For this review, take the finished solid that the model builds, in its own axes (mm). A direction names the side the tool comes from. Give positions to 0.01 mm unless a question says otherwise; leave off trailing zeros. Order: outer loops, then holes, each group sorted by start corner. A loop starts at its lowest first (then second) coordinate and runs counter-clockwise, first axis right, second up. Notation, with made-up numbers: (-33, 79) - (-21, 79) arc R10 cw to (-21, 93) - close; hole circle Ø10 at (21.5, 8). An arc over 180 degrees is marked (long way). Answer as a JSON object with one key per item and string values. Group by question number.
from build123d import *

# Parameters (mm, degrees)
BOSS_EXTRUDE1_DEPTH   = 3
SKETCH2_R             = 6
BOSS_EXTRUDE2_DEPTH   = 4
SKETCH3_R             = 5
BOSS_EXTRUDE3_DEPTH   = 6
SKETCH4_R             = 2.6
CUT_EXTRUDE1_DEPTH    = 20.474342094
SKETCH5_R             = 4
CUT_EXTRUDE2_DEPTH    = 2.5
CUT_EXTRUDE3_START    = -3
SKETCH6_R             = 4
CUT_EXTRUDE3_DEPTH    = 3
M3X0_5_TAPPED_HOLE1_D = 2.5
CHAMFER1_SIZE         = 0.2
FILLET1_R             = 1


with BuildPart() as part:
    # Sketch1 → Boss-Extrude1 (new body)
    with BuildSketch(Plane(origin=(0, 0, 0), x_dir=(1, 0, 0), z_dir=(0, 1, 0))):
        with BuildLine():
            ThreePointArc((-2.104162541, 6.15), (-4.71280541, 4.47654612), (-6.25, 1.785357107))
            ThreePointArc((-6.25, 1.785357107), (-10.5, 0), (-6.25, -1.785357107))
            ThreePointArc((-6.25, -1.785357107), (-4.71280541, -4.47654612), (-2.104162541, -6.15))
            ThreePointArc((-2.104162541, -6.15), (0, -10), (2.104162541, -6.15))
            ThreePointArc((2.104162541, -6.15), (4.71280541, -4.47654612), (6.25, -1.785357107))
            ThreePointArc((6.25, -1.785357107), (10.5, 0), (6.25, 1.785357107))
            ThreePointArc((6.25, 1.785357107), (4.71280541, 4.47654612), (2.104162541, 6.15))
            ThreePointArc((2.104162541, 6.15), (0, 10), (-2.104162541, 6.15))
        make_face()
    extrude(amount=BOSS_EXTRUDE1_DEPTH)

    # Sketch2 → Boss-Extrude2 (add)
    with BuildSketch(Plane(origin=(0, 3, 0), x_dir=(1, 0, 0), z_dir=(0, 1, 0))):
        with Locations(Location((0, 0, 0), (0, 0, 270))):
            Circle(SKETCH2_R)
    extrude(amount=BOSS_EXTRUDE2_DEPTH)

    # Sketch3 → Boss-Extrude3 (add)
    with BuildSketch(Plane(origin=(0, 7, 0), x_dir=(1, 0, 0), z_dir=(0, 1, 0))):
        with Locations(Location((0, 0, 0), (0, 0, 270))):
            Circle(SKETCH3_R)
    extrude(amount=BOSS_EXTRUDE3_DEPTH)

    # Sketch4 → Cut-Extrude1 (cut, through all)
    with BuildSketch(Plane(origin=(0, 13, 0), x_dir=(1, 0, 0), z_dir=(0, 1, 0))):
        with Locations(Location((0, 0, 0), (0, 0, 270))):
            Circle(SKETCH4_R)
    extrude(amount=-CUT_EXTRUDE1_DEPTH, mode=Mode.SUBTRACT)

    # Sketch5 → Cut-Extrude2 (cut)
    with BuildSketch(Plane(origin=(0, 13, 0), x_dir=(1, 0, 0), z_dir=(0, 1, 0))):
        with Locations(Location((0, 0, 0), (0, 0, 270))):
            Circle(SKETCH5_R)
    extrude(amount=-CUT_EXTRUDE2_DEPTH, mode=Mode.SUBTRACT)

    # Sketch6 → Cut-Extrude3 (cut)
    with BuildSketch(Plane.XZ.offset(CUT_EXTRUDE3_START)):
        with Locations(Location((0, 0, 0), (0, 0, 90))):
            Circle(SKETCH6_R)
    extrude(amount=CUT_EXTRUDE3_DEPTH, mode=Mode.SUBTRACT)

    # M3x0.5 Tapped Hole1 (through all)
    with Locations(Plane(origin=(0, 3, 0), x_dir=(1, 0, 0), z_dir=(0, 1, 0))):
        with Locations((0, 7.5), (8, 0), (0, -7.5), (-8, 0)):
            Hole(M3X0_5_TAPPED_HOLE1_D / 2)

    # Chamfer1
    chamfer1_edges = [part.edges().sort_by_distance(p)[0] for p in [
        (0, 13, -5),
    ]]
    chamfer(chamfer1_edges, length=CHAMFER1_SIZE)

    # Fillet1
    fillet1_edges = [part.edges().sort_by_distance(p)[0] for p in [
        (6.25, 1.5, -1.785357107),
        (6.25, 1.5, 1.785357107),
        (2.104162541, 1.5, 6.15),
        (-2.104162541, 1.5, 6.15),
        (-6.25, 1.5, 1.785357107),
        (-6.25, 1.5, -1.785357107),
        (-2.104162541, 1.5, -6.15),
        (2.104162541, 1.5, -6.15),
    ]]
    fillet(fillet1_edges, radius=FILLET1_R)


solid = part.part
1) Consider section C-C (z = -7.5). Give the boundary of the cut face in (x, y), plus the area to 3 significant figures.
2) Mouldability with a two-part tool opening along X and no side actions: class faces 4 (the face through (0.27, 1.48, -6.28)), 5 (the face through (-3.905, 11.768, -0.867)), 6 (the face through (4, 7, -4)), 7 (the face through (4.62, 1.48, 4.57)) as released by +X, released by -X, zero draft, split by the parting line, or undercut.
3) For faces 1 (the face through (0, 10.5, 3)), 2 (the face through (0, 3, 3)), 3 (the face through (10.5, 1.5, 0.1)), list the 3-axis set-ups (+Z, -Z, +X, -X, +Y, -Y) from which the entire face can be reached by the end or side of a thin tool; tool diameter is ignored.
4) Consider section A-A (z = 0). Give the number of separate pieces and of enclosed holes in the cut face, plus the area to 3 significant figures.
5) For pin 1 (2 mm diameter, centred on y = 9, z = -2, fed in from +X); pin 2 (5 mm diameter, centred on y = 11, z = 0, fed in from -X); pin 3 (3 mm diameter, centred on x = -5, y = 6.5, fed in from -Z), all flat-tipped, find the tip position at first contact; note any pin that passes through.
6) Consider section B-B (x = -8). Give the boundary of the cut face in (y, z), plus the area to 3 significant figures.
7) For line 1 (X direction, y = 5, z = 0); line 2 (X direction, y = 1.75, z = -7.5); line 3 (Y direction, x = -3.25, z = -2), list the stretches that pass through material, from the lowest coordinate up.
Result set:
{
 "1": {"outline": "(-2.5, 0) - (-1.25, 0) - (-1.25, 3) - (-2.5, 3) - close; (1.25, 0) - (2.5, 0) - (2.5, 3) - (1.25, 3) - close", "area": "7.50 mm2"},
 "2": {"face 4": "undercut", "face 5": "undercut", "face 6": "zero draft", "face 7": "released by +X"},
 "3": {"face 1": "+Y", "face 2": "-Y", "face 3": "+Y, -Y"},
 "4": {"separate pieces": "4", "enclosed holes": "0", "area": "73.0 mm2"},
 "5": {"pin 1": "stops at x = 4.9", "pin 2": "stops at x = -5", "pin 3": "stops at z = -4.87"},
 "6": {"outline": "(0, -2.5) - (3, -2.5) - (3, -1.25) - (0, -1.25) - close; (0, 1.25) - (3, 1.25) - (3, 2.5) - (0, 2.5) - close", "area": "7.50 mm2"},
 "7": {"line 1": "x = -6 to -2.6, 2.6 to 6", "line 2": "x = -2.5 to -1.25, 1.25 to 2.5", "line 3": "y = 3 to 10.5"}
}
